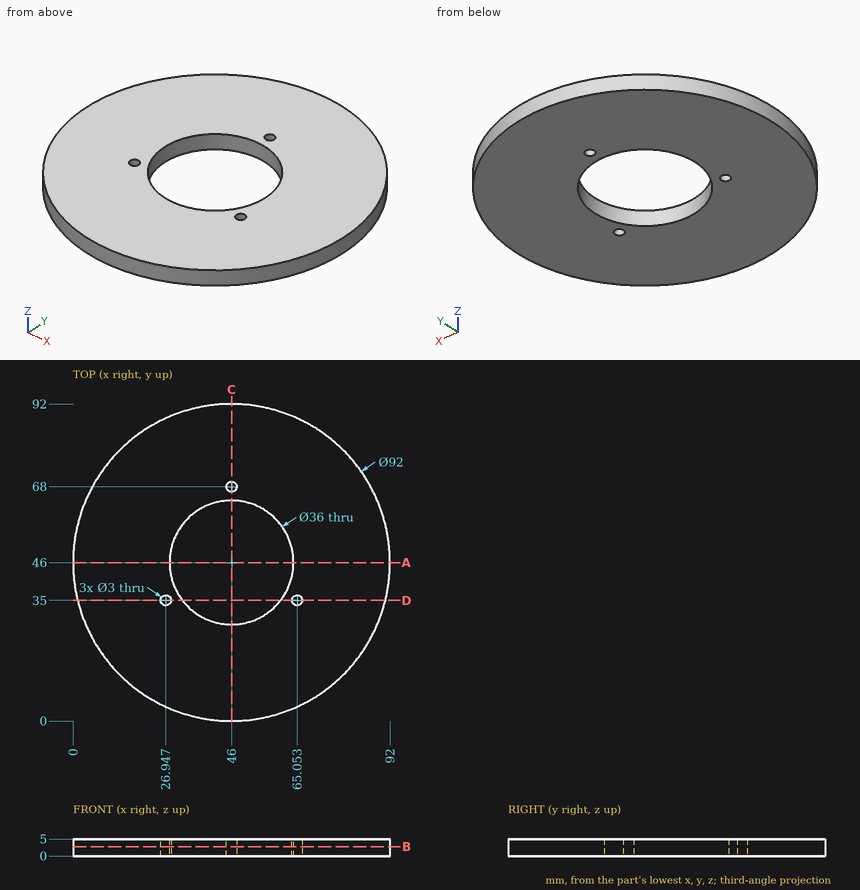
Geometry check sheet. Reference: drawing and pictorial views, mm from the part's lowest x, y, z. Coordinates: 2 decimals unless noted, no trailing zeros. Order: outer loops, then holes, each group sorted by start corner. A loop starts at its lowest first (then second) coordinate and runs counter-clockwise, first axis right, second up. Notation, with made-up numbers: M 29.25,21 L 48.25,21 A24 cw 48.25,35 Z; hole C 18,77.25 d7. An arc over 180 degrees is marked long. Return JSON: item names as keys, results as strings.
1) Gauge pin test, flat ends, axial feed: pin 1 (1.5 mm diameter, centred on x = 24.5, z = 2, fed in from +Y) (1 decimal); pin 2 (1.5 mm diameter, centred on y = 61.5, z = 3.5, fed in from +X); pin 3 (1 mm diameter, centred on x = 41, z = 1, fed in from +Y). Record the tip position at first contact, or that the pin passes through.
Answer list:
{"pin 1": "y = 87.1", "pin 2": "x = 89.57", "pin 3": "y = 91.78"}
2) Cross-section at C-C, the plane x = 46. Record the boundary of the cut face in (y, z).
Answer list:
{"outline": "M 0,0 L 28,0 L 28,5 L 0,5 Z; M 64,0 L 66.5,0 L 66.5,5 L 64,5 Z; M 69.5,0 L 92,0 L 92,5 L 69.5,5 Z"}
3) Cross-section at B-B, the plane z = 2.8. Record the boundary of the cut face in (x, y), and give its area (3 significant figures).
Answer list:
{"outline": "C 46,46 d92; hole C 26.95,35 d3; hole C 46,46 d36; hole C 46,68 d3; hole C 65.05,35 d3", "area": "5,610 mm2"}
4) Thickness scan on L1, parallel to Y at x = 46, z = 2.5; L2, parallel to X at y = 68, z = 2.35; L3, parallel to Y at x = 66, z = 3 (1 decimal). Record the ranges inside material, lowest first. Write a range as [from, to].
Answer list:
{"L1": "[0, 28], [64, 66.5], [69.5, 92]", "L2": "[5.6, 44.5], [47.5, 86.4]", "L3": "[4.6, 33.8], [36.2, 87.4]"}
5) Cross-section at A-A, the plane y = 46. Record the boundary of the cut face in (x, z).
Answer list:
{"outline": "M 0,0 L 28,0 L 28,5 L 0,5 Z; M 64,0 L 92,0 L 92,5 L 64,5 Z"}
6) Cross-section at D-D, the plane y = 35. Record the boundary of the cut face in (x, z) (1 decimal), and give its area (3 significant figures).
Answer list:
{"outline": "M 1.3,0 L 25.4,0 L 25.4,5 L 1.3,5 Z; M 28.4,0 L 31.8,0 L 31.8,5 L 28.4,5 Z; M 60.2,0 L 63.6,0 L 63.6,5 L 60.2,5 Z; M 66.6,0 L 90.7,0 L 90.7,5 L 66.6,5 Z", "area": "274 mm2"}
